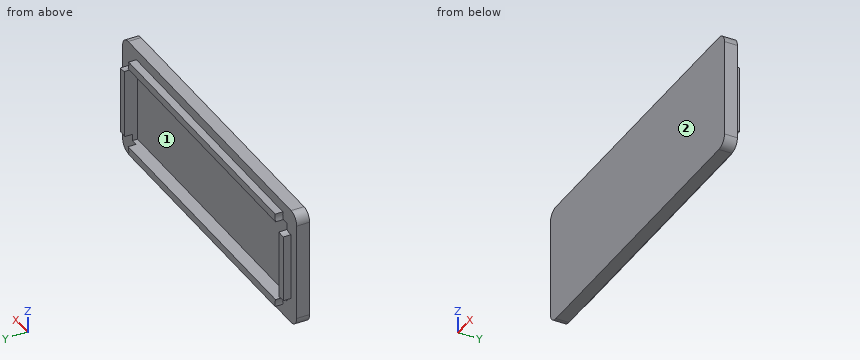
```python
from build123d import *

# Parameters (mm, degrees)
F0_W     = 62.5
F0_H     = 23
F1_DEPTH = 2.5
F2_T     = -2
F3_R     = 2
F4_DEPTH = 2
F5_T     = -1.5
F6_R     = 2.5
F7_DEPTH = 2


# Not quite as in the source:
# - a feature names something its author has since deleted; it is built from what else it names


with BuildPart() as f1:
    # F0 (on Front) → F1 (new body)
    with BuildSketch(Plane.XZ):
        Rectangle(F0_W, F0_H)
    extrude(amount=F1_DEPTH)

    # F2
    f2_openings = [f1.faces().sort_by_distance(p)[0] for p in [
        (0, 0, 0),
    ]]
    offset(amount=F2_T, openings=f2_openings)

    # F3
    f3_edges = [f1.edges().sort_by_distance(p)[0] for p in [
        (-31.25, -1.25, 11.5),
        (-31.25, -1.25, -11.5),
        (31.25, -1.25, 11.5),
        (31.25, -1.25, -11.5),
    ]]
    fillet(f3_edges, radius=F3_R)

    # F4 (add): a face of the model
    f4_faces = [f1.faces().sort_by_distance(p)[0] for p in [
        (0, -0.5, 0),
    ]]
    extrude(f4_faces, amount=F4_DEPTH)

    # F5
    f5_openings = [f1.faces().sort_by_distance(p)[0] for p in [
        (0, 1.5, 0),
    ]]
    offset(amount=F5_T, openings=f5_openings, kind=Kind.INTERSECTION)

    # F6 (on face) → F7 (cut)
    with BuildSketch(Plane(origin=(0, 0, 0), x_dir=(-1, 0, 0), z_dir=(0, 1, 0))):
        with Locations((-28.75, 9)):
            Circle(F6_R)
        with Locations((28.75, 9)):
            Circle(F6_R)
        with Locations((28.75, -9)):
            Circle(F6_R)
        with Locations((-28.75, -9)):
            Circle(F6_R)
    extrude(amount=F7_DEPTH, mode=Mode.SUBTRACT)


solid = f1.part
```
Geometry: final body of the model. Coordinates: model frame, mm. Face numbers are marked on the shaded views. Coordinates: 2 decimals unless noted, no trailing zeros. Order: outer loops, then holes, each group sorted by start corner. A loop starts at its lowest first (then second) coordinate and runs counter-clockwise, first axis right, second up. Notation, with made-up numbers: M 75.5,-11 L 106.5,-11 A9 cw 106.5,4 Z; hole C 14.5,-32.5 d11. An arc over 180 degrees is marked long. Answer as CSV lines item,"result".
Q1. First-contact query: P1, Ø8, axis at x = -7.5, z = -7.5, coming from the +Y side; P2, Ø8, axis at x = -10.5, z = 0, coming from the +Y side; P3, Ø1.2, axis at y = 1, z = -1, coming from the -X side; P4, Ø0.8, axis at x = -2, y = 1, coming from the +Z side. Flat tips, straight axial feed; report the tip coordinate or a pass-through.
Answers:
P1,"stops at y = 1.5"
P2,"stops at y = -1"
P3,"stops at x = -29.25"
P4,"stops at z = 9.5"
Q2. Section B-B on x = 8. Return the cut outline in (y, z), and give its area (3 significant figures).
Answers:
outline,"M -2.5,-11.5 L 0,-11.5 L 0,-9.5 L 1.5,-9.5 L 1.5,-8 L -1,-8 L -1,8 L 1.5,8 L 1.5,9.5 L 0,9.5 L 0,11.5 L -2.5,11.5 Z"
area,"46.0 mm^2"
Q3. Line query: probe 1 along Z at (x, y) = (-3, 1.05); probe 2 along X at (y, z) = (0.8, -0.5); probe 3 along Z at (x, y) = (3, -0.1). Output: solid intervals per line, ascending. Write a range as [from, to].
Answers:
probe 1,"z = [-9.5, -8], [8, 9.5]"
probe 2,"x = [-29.25, -27.75], [27.75, 29.25]"
probe 3,"z = [-11.5, -8], [8, 11.5]"
Q4. Draft query along Y for the marked faces 1 and 2. Return one class per face: pulls with the +Y half, pulls with the -Y half, needs draft (parallel to the pull), parting line crosses it, or undercut.
Answers:
face 1,"pulls with the +Y half"
face 2,"pulls with the -Y half"
Q5. Section A-A on z = 3. Return the cut outline in (x, y), and give its area (3 significant figures).
Answers:
outline,"M -31.25,-2.5 L 31.25,-2.5 L 31.25,0 L 29.25,0 L 29.25,1.5 L 27.75,1.5 L 27.75,-1 L -27.75,-1 L -27.75,1.5 L -29.25,1.5 L -29.25,0 L -31.25,0 Z"
area,"105 mm^2"
